The model under review builds one solid part; all positions refer to its coordinate system, in mm. Face numbers are marked on the shaded views. A direction names the side the tool comes from. Give positions to 0.01 mm unless a question says otherwise; leave off trailing zeros. Loops run counter-clockwise (first coordinate to the right, second up) from the corner with the lowest first, then second, coordinate; pieces in that order, holes last. Notation, with made-up numbers: (-14.75, -13.75) - (6.25, -13.75) arc R21 ccw to (6.25, 8.25) - close; hole circle Ø3 at (-18.75, -6). An arc over 180 degrees is marked (long way). Answer as a JSON object with one key per item and string values.
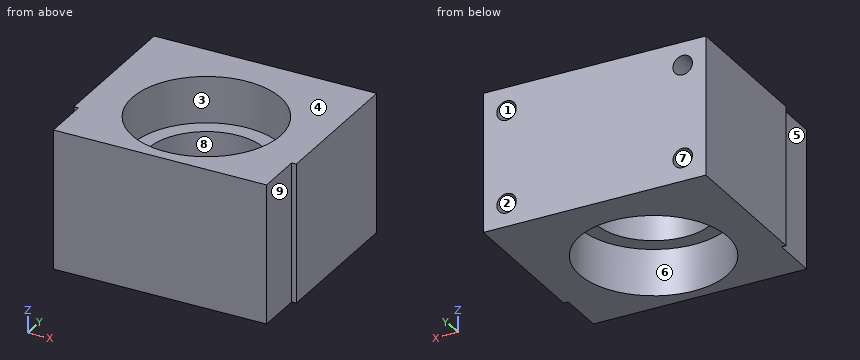
from build123d import *

# Parameters (mm, degrees)
SZKIC1_W                       = 48
SZKIC1_H                       = 30
DODANIE_WYCI_GNI_CIE1_DEPTH    = 42
SZKIC3_R                       = 12.5
WYTNIJ_WYCI_GNI_CIE2_DEPTH     = 57.920997883
SZKIC4_R                       = 16
WYTNIJ_WYCI_GNI_CIE3_DEPTH     = 10
OTW_R_GWINTOWANY_M5X0_81_D     = 4.2
OTW_R_GWINTOWANY_M5X0_81_DEPTH = 35
OTW_R_GWINTOWANY_M5X0_81_TIP   = 1.2618073
SZKIC10_W                      = 1
SZKIC10_H                      = 10
WYTNIJ_WYCI_GNI_CIE4_DEPTH     = 57.920997883


with BuildPart() as part:
    # Szkic1 → Dodanie-wyciągnięcie1 (new body)
    with BuildSketch(Plane(origin=(0, 0, 0), x_dir=(1, 0, 0), z_dir=(0, 1, 0))):
        Rectangle(SZKIC1_W, SZKIC1_H)
    extrude(amount=DODANIE_WYCI_GNI_CIE1_DEPTH)

    # Szkic3 → Wytnij-wyciągnięcie2 (cut, through all)
    with BuildSketch(Plane.XY.offset(15)):
        with Locations((0, 18.5)):
            Circle(SZKIC3_R)
    extrude(amount=-WYTNIJ_WYCI_GNI_CIE2_DEPTH, mode=Mode.SUBTRACT)

    # Szkic4 → Wytnij-wyciągnięcie3 (cut)
    with BuildSketch(Plane.XY.offset(15)):
        with Locations((0, 18.5)):
            Circle(SZKIC4_R)
    wytnij_wyci_gni_cie3 = extrude(amount=-WYTNIJ_WYCI_GNI_CIE3_DEPTH, mode=Mode.SUBTRACT)

    # Lustro1: Wytnij-wyciągnięcie3 across plane
    add(wytnij_wyci_gni_cie3.mirror(Plane.XY), mode=Mode.SUBTRACT)

    # Otwór gwintowany M5x0.81
    with Locations(Plane(origin=(0, 42, 0), x_dir=(1, 0, 0), z_dir=(0, 1, 0))):
        with Locations((-19, -10), (-19, 10), (19, -10), (19, 10)):
            Hole(OTW_R_GWINTOWANY_M5X0_81_D / 2, depth=OTW_R_GWINTOWANY_M5X0_81_DEPTH)
            with Locations((0, 0, -(OTW_R_GWINTOWANY_M5X0_81_DEPTH + OTW_R_GWINTOWANY_M5X0_81_TIP / 2))):  # 118° drill point
                Cone(0, OTW_R_GWINTOWANY_M5X0_81_D / 2, OTW_R_GWINTOWANY_M5X0_81_TIP, mode=Mode.SUBTRACT)

    # Szkic10 → Wytnij-wyciągnięcie4 (cut, through all)
    with BuildSketch(Plane.XY.offset(15)):
        with Locations((23.5, 5)):
            Rectangle(SZKIC10_W, SZKIC10_H)
        with Locations((-23.5, 5)):
            Rectangle(SZKIC10_W, SZKIC10_H)
    extrude(amount=-WYTNIJ_WYCI_GNI_CIE4_DEPTH, mode=Mode.SUBTRACT)


solid = part.part
Q1. Clearance check with flat-ended pins moving along their axes: pin 1 Ø5.5 at (x, z) = (19, 10) entering from +Y; pin 2 Ø0.5 at (x, z) = (-23.5, 3.5) entering from -Y; pin 3 Ø5 at (y, z) = (2.5, 4.5) entering from -X; pin 4 Ø4 at (x, z) = (-19, -10) entering from +Y. State where each tip first meets the part, or that it passes through.
Results:
{"pin 1": "stops at y = 42", "pin 2": "stops at y = 10", "pin 3": "stops at x = -23", "pin 4": "stops at y = 6.94"}
Q2. To check wall thickness, follow probe 1 along Z at (x, y) = (-19, 18); probe 2 along Z at (x, y) = (17.5, 14.5); probe 3 along X at (y, z) = (25, -9.75). State the ranges of each line that lie inside material, in increasing order. Write a range as [from, to].
Results:
{"probe 1": "z = [-15, -12.1], [-7.9, 7.9], [12.1, 15]", "probe 2": "z = [-15, -11.47], [-8.53, 8.53], [11.47, 15]", "probe 3": "x = [-24, -21.09], [-16.91, -14.62], [14.62, 16.91], [21.09, 24]"}
Q3. Consider section B-B, the plane x = 0. State the section outline as (y, z) points.
Results:
{"outline": "(0, -15) - (2.5, -15) - (2.5, -5) - (6, -5) - (6, 5) - (2.5, 5) - (2.5, 15) - (0, 15) - close; (31, -5) - (34.5, -5) - (34.5, -15) - (42, -15) - (42, 15) - (34.5, 15) - (34.5, 5) - (31, 5) - close"}
Q4. Consider section D-D, the plane y = 37. State the section outline as (x, z) points.
Results:
{"outline": "(-24, -15) - (24, -15) - (24, 15) - (-24, 15) - close; hole circle Ø4.2 at (-19, -10); hole circle Ø4.2 at (-19, 10); hole circle Ø4.2 at (19, -10); hole circle Ø4.2 at (19, 10)"}
Q5. Consider section A-A, the plane y = 18.5. State the section outline as (x, z) points, plus the area to 3 significant figures.
Results:
{"outline": "(-24, -15) - (-16, -15) - (-16, -5) - (-12.5, -5) - (-12.5, 5) - (-16, 5) - (-16, 15) - (-24, 15) - close; (12.5, -5) - (16, -5) - (16, -15) - (24, -15) - (24, 15) - (16, 15) - (16, 5) - (12.5, 5) - close; hole circle Ø4.2 at (-19, -10); hole circle Ø4.2 at (-19, 10); hole circle Ø4.2 at (19, -10); hole circle Ø4.2 at (19, 10)", "area": "495 mm^2"}
Q6. Consider section C-C, the plane z = 3. State the section outline as (x, y) points, plus the area to 3 significant figures.
Results:
{"outline": "(-24, 10) - (-23, 10) - (-23, 0) - (23, 0) - (23, 10) - (24, 10) - (24, 42) - (-24, 42) - close; hole circle Ø25 at (0, 18.5)", "area": "1,510 mm^2"}
Q7. For the marked faces 5, 6, 7, 8 and 9, list the 3-axis set-ups (+Z, -Z, +X, -X, +Y, -Y) from which the entire face can be reached by the end or side of a thin tool; tool diameter is ignored.
Results:
{"face 5": "+Z, -Z, -X, -Y", "face 6": "-Z", "face 7": "+Y", "face 8": "+Z, -Z", "face 9": "+Z, -Z, +X, -Y"}
Q8. The part is to be moulded in two halves that separate along Z. For the marked faces 1, 2, 3 and 4, say which applies: +Z half, -Z half, draft (parallel to the pull), parting line (faces both ways), or undercut.
Results:
{"face 1": "undercut", "face 2": "undercut", "face 3": "draft", "face 4": "+Z half"}
